```python
from build123d import *


with BuildPart() as part:
    # Sketch1 → Revolve1 (revolve)
    with BuildSketch(Plane(origin=(0, 0, 0), x_dir=(0, 0, -1), z_dir=(1, 0, 0)), mode=Mode.PRIVATE) as revolve1_sk:
        with BuildLine():
            Line((0, 0), (3, 0))
            ThreePointArc((3, 0), (2.938994507, 2.469175495), (2.756126895, 4.932325659))
            Line((2.756126895, 4.932325659), (2.506126895, 4.932325659))
            Line((2.506126895, 4.932325659), (2, 4.95))
            Line((2, 4.95), (2, 5))
            Line((2, 5), (0.22651456, 5))
            ThreePointArc((0.22651456, 5), (0.157503692, 4.979613789), (0.110648258, 4.925))
            Line((0.110648258, 4.925), (0.060648258, 4.925))
            ThreePointArc((0.060648258, 4.925), (0.015162639, 2.462686704), (0, 0))
        make_face()
    revolve(revolve1_sk.sketch.rotate(Axis((0, 0, -7.414080755), (0, 0, 1)), 90), axis=Axis((0, 0, -7.414080755), (0, 0, 1)))


solid = part.part
```
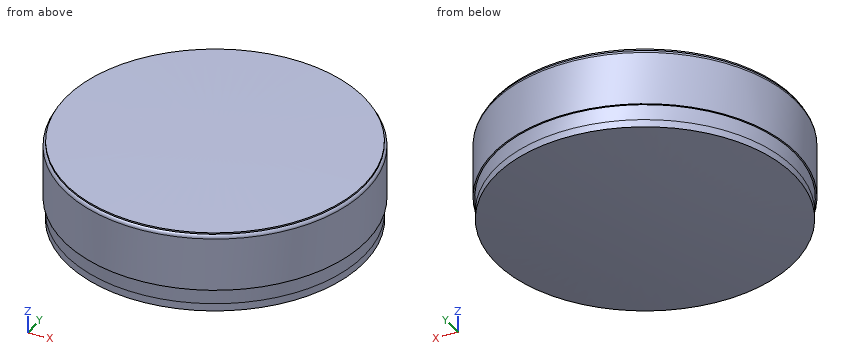
The model under review builds one solid part; all positions refer to its coordinate system, in mm. Give positions to 0.01 mm unless a question says otherwise; leave off trailing zeros. Write each loop counter-clockwise with the first axis right and the second up, starting at its lowest first coordinate (ties: lowest second). Pieces come first, ordered by that corner, then holes. Notation, with made-up numbers: (72, 60) - (119, 60) arc R36 cw to (119, 95) - close; hole circle Ø10 at (16.5, -16.75). An arc over 180 degrees is marked (long way). Answer in a Markdown table with one row per item. Add a question column.
1. Insertion check: P1, Ø1, axis at x = -4, y = -3.5, coming from the +Z side; P2, Ø1.5, axis at x = 1.5, y = -1, coming from the -Z side; P3, Ø1, axis at x = 3.5, z = -0.5, coming from the -Y side. Each pin has a flat end and moves straight along its axis. Give the tip position at first contact, or say it passes through.
2. Wall thickness on line 1 along X through (y, z) = (-4.5, -2.1); line 2 along X through (y, z) = (3, -2.05); line 3 along Y through (x, z) = (-1, -1.9): over which ranges is each line inside the solid? List them lowest first. Write a range as [from, to].
3. We need section A-A on x = 0. Write out the cut boundary in (y, z) (3 decimals), then the cut area to 3 significant figures.
4. We need section C-C on z = -1.2. Write out the cut boundary in (x, y), then the cut area to 3 significant figures.
Ans:
| question | item | result |
|---|---|---|
| 1 | P1 | stops at z = -0.06 |
| 1 | P2 | stops at z = -2.99 |
| 1 | P3 | stops at y = -4 |
| 2 | line 1 | x = [-2.05, 2.05] |
| 2 | line 2 | x = [-3.94, 3.94] |
| 2 | line 3 | y = [-4.9, 4.9] |
| 3 | outline | (-5, -2) - (-4.95, -2) - (-4.932, -2.506) - (-4.932, -2.756) arc R50 ccw to (4.932, -2.756) - (4.932, -2.506) - (4.95, -2) - (5, -2) - (5, -0.227) arc R0.127 ccw to (4.925, -0.111) - (4.925, -0.061) arc R200 ccw to (-4.925, -0.061) - (-4.925, -0.111) arc R0.127 ccw to (-5, -0.227) - close |
| 3 | area | 28.9 mm^2 |
| 4 | outline | circle Ø10 at (0, 0) |
| 4 | area | 78.5 mm^2 |
